```python
from build123d import *

# Parameters (mm, degrees)
SKETCH_6_R          = 1.984
EXTRUDE_2_DEPTH     = 6.35
SKETCH_7_W          = 6.35
SKETCH_7_H          = 28
EXTRUDE_3_DEPTH     = 60
SKETCH_8_W          = 4
SKETCH_8_H          = 5
SKETCH_8_H_2        = 4.5
CUT_EXTRUDE_3_DEPTH = 250


with BuildPart() as part:
    # 草图6 → 凸台-拉伸2 (new body)
    with BuildSketch(Plane(origin=(0, 3, 0), x_dir=(1, 0, 0), z_dir=(0, 1, 0))):
        Polygon((98.316405333, 0), (91.966405333, 0), (80.5, 0), (64.197651568, 46.16), (-64.197651568, 46.16), (-80.5, 0), (-91.966405333, 0), (-98.316405333, 0), (-98.316405333, 120.32), (-91.966405333, 120.32), (-80.5, 74.16), (-64.197651568, 74.16), (64.197651568, 74.16), (80.5, 74.16), (91.966405333, 120.32), (98.316405333, 120.32), align=None)
        with Locations((91.966405333, 12.7)):
            Circle(SKETCH_6_R, mode=Mode.SUBTRACT)
        with Locations((91.966405333, 107.62)):
            Circle(SKETCH_6_R, mode=Mode.SUBTRACT)
        with Locations((-91.966405333, 12.7)):
            Circle(SKETCH_6_R, mode=Mode.SUBTRACT)
        with Locations((-91.966405333, 107.62)):
            Circle(SKETCH_6_R, mode=Mode.SUBTRACT)
    extrude(amount=EXTRUDE_2_DEPTH)

    # 草图7 → 凸台-拉伸3 (add)
    with BuildSketch(Plane(origin=(0, 9.35, 0), x_dir=(1, 0, 0), z_dir=(0, 1, 0))):
        with Locations((84.175, 60.16)):
            Rectangle(SKETCH_7_W, SKETCH_7_H)
        with Locations((-84.175, 60.16)):
            Rectangle(SKETCH_7_W, SKETCH_7_H)
    extrude(amount=EXTRUDE_3_DEPTH)

    # 草图8 → 切除-拉伸3 (cut)
    with BuildSketch(Plane(origin=(87.35, 0, 0), x_dir=(0, 0, -1), z_dir=(1, 0, 0))):
        with Locations((50.49, 65.44)):
            Rectangle(SKETCH_8_W, SKETCH_8_H)
        with Locations((60.31, 65.44)):
            Rectangle(SKETCH_8_W, SKETCH_8_H)
        with Locations((70.13, 65.19)):
            Rectangle(SKETCH_8_W, SKETCH_8_H_2)
    extrude(amount=-CUT_EXTRUDE_3_DEPTH, mode=Mode.SUBTRACT)


solid = part.part
```
Part model, mm, in its own coordinate system. A direction names the side the tool comes from. Round coordinates to 2 decimals unless told otherwise and drop trailing zeros. Order: outer loops, then holes, each group sorted by start corner. A loop starts at its lowest first (then second) coordinate and runs counter-clockwise, first axis right, second up. Notation, with made-up numbers: M 88,22.5 L 133,22.5 A24 cw 133,34.5 Z; hole C 40,-19 d6. An arc over 180 degrees is marked long. Answer in a Markdown table with one row per item. Add a question column.
Q1. Cut at D-D on x = -58. Give the cut face in (y, z), and give its area (3 significant figures).
Q2. Cut at C-C on z = -92. Give the cut face in (x, y).
Q3. Pin check, flat tips, straight feed: pin 1 (10 mm diameter, centred on y = 50.5, z = -76, fed in from +X); pin 2 (12 mm diameter, centred on x = 60.5, z = -80, fed in from +Y); pin 3 (5 mm diameter, centred on x = -85, y = 64, fed in from -Z); pin 4 (2 mm diameter, centred on y = 12, z = -107.5, fed in from -X). Stop position of each tip, or through.
Q4. Cut at A-A on z = -12.7. Give the cut face in (x, y), and give its area (3 significant figures).
Q5. Mould opens along Y. For faces 1 (the face through (-84, 69.35, -60)), 2 (the face through (-90, 6, 0)), 3 (the face through (-84, 65, -52.49)) say: +Y half, -Y half, draft (parallel to the pull), parting line (faces both ways), or undercut.
Q6. 3-axis set-ups, long thin cutter, end or side, ignore diameter. For faces 4 (the face through (1, 6, -74.16)), 5 (the face through (-84, 39, -46.16)), 6 (the face through (-84, 67.44, -70)): which of +Z, -Z, +X, -X, +Y, -Y reach the whole face in a straight line?
Q7. Cut at B-B on y = 24. Give the cut face in (x, z).
Q8. Wall check: L1, parallel to X at y = 47, z = -51.5; L2, parallel to X at y = 4.5, z = -107.62; L3, parallel to X at y = 6, z = -12. Give the ranges that are in metal, low to high. Write a range as from..to.
Established:
| question | item | result |
|---|---|---|
| 1 | outline | M 3,-74.16 L 9.35,-74.16 L 9.35,-46.16 L 3,-46.16 Z |
| 1 | area | 178 mm2 |
| 2 | outline | M -98.32,3 L -84.93,3 L -84.93,9.35 L -98.32,9.35 Z; M 84.93,3 L 98.32,3 L 98.32,9.35 L 84.93,9.35 Z |
| 3 | pin 1 | stops at x = 87.35 |
| 3 | pin 2 | stops at y = 9.35 |
| 3 | pin 3 | stops at z = -74.16 |
| 3 | pin 4 | passes through |
| 4 | outline | M -98.32,3 L -93.95,3 L -93.95,9.35 L -98.32,9.35 Z; M -89.98,3 L -76.01,3 L -76.01,9.35 L -89.98,9.35 Z; M 76.01,3 L 89.98,3 L 89.98,9.35 L 76.01,9.35 Z; M 93.95,3 L 98.32,3 L 98.32,9.35 L 93.95,9.35 Z |
| 4 | area | 233 mm2 |
| 5 | face 1 | +Y half |
| 5 | face 2 | draft |
| 5 | face 3 | undercut |
| 6 | face 4 | -Z, +Y, -Y |
| 6 | face 5 | +Z, +X, -X, +Y |
| 6 | face 6 | +X, -X |
| 7 | outline | M -87.35,-74.16 L -81,-74.16 L -81,-46.16 L -87.35,-46.16 Z; M 81,-74.16 L 87.35,-74.16 L 87.35,-46.16 L 81,-46.16 Z |
| 8 | L1 | x = -87.35..-81, 81..87.35 |
| 8 | L2 | x = -98.32..-93.95, -89.98..-88.81, 88.81..89.98, 93.95..98.32 |
| 8 | L3 | x = -98.32..-93.82, -90.11..-76.26, 76.26..90.11, 93.82..98.32 |
